```python
from build123d import *

# Parameters (mm, degrees)
SKETCH2_R           = 3.5
BOSS_EXTRUDE1_DEPTH = 15
SKETCH3_R           = 2.75
CUT_EXTRUDE1_DEPTH  = 15
SKETCH4_R           = 2.75
CUT_EXTRUDE2_DEPTH  = 15
FILLET1_R           = 5
FILLET2_R           = 1


with BuildPart() as part:
    # Sketch2 → Boss-Extrude1 (new body)
    with BuildSketch(Plane(origin=(0, 0, 0), x_dir=(0, 0, -1), z_dir=(1, 0, 0))):
        Polygon((0, 3.386529676), (0, 40), (7.5, 40), (7.5, 28), (28, 7.5), (40, 7.5), (40, 0), (3.386529676, 0), align=None)
        with Locations((10, 10)):
            Circle(SKETCH2_R, mode=Mode.SUBTRACT)
    extrude(amount=BOSS_EXTRUDE1_DEPTH)

    # Sketch3 → Cut-Extrude1 (cut)
    with BuildSketch(Plane(origin=(0, 7.5, 0), x_dir=(1, 0, 0), z_dir=(0, 1, 0))):
        with Locations(Location((7.5, 34, 0), (0, 0, 270))):
            Circle(SKETCH3_R)
    extrude(amount=-CUT_EXTRUDE1_DEPTH, mode=Mode.SUBTRACT)

    # Sketch4 → Cut-Extrude2 (cut)
    with BuildSketch(Plane(origin=(0, 0, -7.5), x_dir=(-1, 0, 0), z_dir=(0, 0, -1))):
        with Locations(Location((-7.5, 34, 0), (0, 0, 90))):
            Circle(SKETCH4_R)
    extrude(amount=-CUT_EXTRUDE2_DEPTH, mode=Mode.SUBTRACT)

    # Fillet1
    fillet1_edges = [part.edges().sort_by_distance(p)[0] for p in [
        (7.5, 28, -7.5),
        (7.5, 7.5, -28),
    ]]
    fillet(fillet1_edges, radius=FILLET1_R)

    # Fillet2
    fillet2_edges = [part.edges().sort_by_distance(p)[0] for p in [
        (7.5, 40, -7.5),
        (7.5, 7.5, -40),
    ]]
    fillet(fillet2_edges, radius=FILLET2_R)


solid = part.part
```
Can you work these out from the model? Positions are in its coordinate system, mm. A direction names the side the tool comes from. Coordinates: 2 decimals unless noted, no trailing zeros. Write each loop counter-clockwise with the first axis right and the second up, starting at its lowest first coordinate (ties: lowest second). Pieces come first, ordered by that corner, then holes. Notation, with made-up numbers: M 22.25,-34 L 40.25,-34 A15 ccw 40.25,-27 Z; hole C 37.5,47.25 d2. An arc over 180 degrees is marked long. Write item = value, one per line. Start each with the question number.
Q1. If I drill on L1, parallel to X at y = 34, z = -5; L2, parallel to Z at x = 3.75, y = 31; L3, parallel to Y at x = 5, z = -10, over which ranges is the centre line in solid material (lowest first)? Write a range as [from, to].
Q2. If we section it at A-A, the plane x = 7.5: Write out the boundary of the cut face in (y, z), then the cut area to 3 significant figures.
Q3. On a 3-axis mill with a long thin cutter (end or side, diameter ignored), from which of +Z, -Z, +X, -X, +Y, -Y can I reach the whole of each face in a straight line? I mean faces 4 (the face through (9, 37, -7.5)), 5 (the face through (7, 0, -22)). Say none if no direction works.
Q4. If we section it at C-C, the plane z = -10: Write out the boundary of the cut face in (x, y).
Q5. Thinking about a two-plate mould opening in Z: for faces 1 (the face through (7, 3, -40)), 2 (the face through (7.4, 7.9, -7.2)), 3 (the face through (15, 16, -16)), which applies, released by +Z, released by -Z, zero draft, split by the parting line, or undercut?
Q6. If we section it at B-B, the plane y = 34: Write out the boundary of the cut face in (x, z).
Q7. If we section it at D-D, the plane y = 7: Write out the boundary of the cut face in (x, z).
Check sheet entries:
q1.L1 = [0, 4.75], [10.25, 15]
q1.L2 = [-7.5, 0]
q1.L3 = [0, 6.5], [13.5, 25.5]
q2.outline = M 0,-40 L 6.5,-40 A1 ccw 7.5,-39 L 7.5,-36.75 L 0,-36.75 Z; M 0,-31.25 L 7.5,-31.25 L 7.5,-30.07 A5 cw 8.96,-26.54 L 26.54,-8.96 A5 cw 30.07,-7.5 L 31.25,-7.5 L 31.25,0 L 3.39,0 L 0,-3.39 Z; M 36.75,-7.5 L 39,-7.5 A1 ccw 40,-6.5 L 40,0 L 36.75,0 Z; hole C 10,-10 d7
q2.area = 628 mm²
q3.face_4 = -Z, +X, -X, +Y
q3.face_5 = +Z, -Z, +X, -X, -Y
q4.outline = M 0,0 L 15,0 L 15,6.5 L 0,6.5 Z; M 0,13.5 L 15,13.5 L 15,25.5 L 0,25.5 Z
q5.face_1 = released by -Z
q5.face_2 = undercut
q5.face_3 = zero draft
q6.outline = M 0,-7.5 L 4.75,-7.5 L 4.75,0 L 0,0 Z; M 10.25,-7.5 L 15,-7.5 L 15,0 L 10.25,0 Z
q7.outline = M 0,-39.87 L 15,-39.87 L 15,-11.8 L 0,-11.8 Z; M 0,-8.2 L 15,-8.2 L 15,0 L 0,0 Z; hole C 7.5,-34 d5.5
